from build123d import *

# Parameters (mm, degrees)
F0_W      = 5
F0_H      = 20
F1_DEPTH  = 35
F2_W      = 90
F2_H      = 25
F3_DEPTH  = 79.8669262783
F4_W      = 20
F4_H      = 35.1404882967
F5_DEPTH  = 5
F6_W      = 60
F6_H      = 25
F7_DEPTH  = 8.9178062806
F8_W      = 8.9168062806
F8_H      = 25
F9_DEPTH  = 12.5
F10_W     = 0.6563552694
F10_H     = 25
F11_DEPTH = 5
F12_W     = 7.5
F12_H     = 10
F13_DEPTH = 10


with BuildPart() as f1:
    # F0 (on Top) → F1 (new body)
    with BuildSketch(Plane.XY):
        Polygon((1.4652782414, 46.6247905791), (-88.5347217586, 60), (-88.5347217586, 40), (-88.5347217586, 0), (-88.5347217586, -20), (1.4652782414, -13.3752094209), align=None)
        with Locations((-91.0347217586, 50)):
            Rectangle(F0_W, F0_H)
        with Locations((-91.0347217586, -10)):
            Rectangle(F0_W, F0_H)
    extrude(amount=F1_DEPTH)

    # F2 (on face) → F3 (cut, through all)
    with BuildSketch(Plane(origin=(6.8110049505, 45.8303437542, 0), x_dir=(-0.9891366412, 0.1469989969, 0), z_dir=(0.1469989969, 0.9891366412, 0))):
        with Locations((50.404437048, 17.5)):
            Rectangle(F2_W, F2_H)
    extrude(amount=-F3_DEPTH, mode=Mode.SUBTRACT)

    # F4 (on face) → F5 (join)
    with BuildSketch(Plane(origin=(-93.5347217586, 0, 0), x_dir=(0, -1, 0), z_dir=(-1, 0, 0))):
        with Locations((10, 17.5702441484)):
            Rectangle(F4_W, F4_H)
    extrude(amount=-F5_DEPTH)

    # F6 (on face) → F7 (cut, through all)
    with BuildSketch(Plane.YZ.offset(1.4652782414)):
        with Locations((16.6247905791, 17.5)):
            Rectangle(F6_W, F6_H)
    extrude(amount=-F7_DEPTH, mode=Mode.SUBTRACT)

    # F8 (on face) → F9 (cut, symmetric)
    with BuildSketch(Plane(origin=(0, -13.3752094209, 0), x_dir=(-1, 0, 0), z_dir=(0, 1, 0))):
        with Locations((2.9931248989, 17.5)):
            Rectangle(F8_W, F8_H)
    extrude(amount=F9_DEPTH, both=True, mode=Mode.SUBTRACT)

    # F10 (on face) → F11 (cut, symmetric)
    with BuildSketch(Plane.YZ.offset(-7.4515280392)):
        with Locations((-13.7033870556, 17.5)):
            Rectangle(F10_W, F10_H)
    extrude(amount=F11_DEPTH, both=True, mode=Mode.SUBTRACT)

    # F12 (on face) → F13 (join)
    with BuildSketch(Plane.XY.offset(35)):
        with Locations((-64.7847217586, 25)):
            Rectangle(F12_W, F12_H)
    extrude(amount=F13_DEPTH)


solid = f1.part
The model under review builds one solid part; all positions refer to its coordinate system, in mm. A direction names the side the tool comes from. Round coordinates to 2 decimals unless told otherwise and drop trailing zeros. Write each loop counter-clockwise with the first axis right and the second up, starting at its lowest first coordinate (ties: lowest second). Pieces come first, ordered by that corner, then holes. Notation, with made-up numbers: M 9.25,80.5 L 45.25,80.5 A24 ccw 45.25,114.5 Z; hole C 68.25,55 d10. An arc over 180 degrees is marked long. Use a Markdown table: item, result. Add a question column.
Q1. Machinability: for faces 5 (the face through (-93.535, -10, 17)), 6 (the face through (-88.535, 20, 32)), 7 (the face through (-61.035, 25, 40)), which of the approach directions +Z, -Z, +X, -X, +Y, -Y give a long, thin tool a straight path to every point of the face, cutting with its end or side? Answer none if there is none.
Q2. We need section D-D, the plane y = -10. State the section outline as (x, z) points.
Q3. To check wall thickness, follow line 1 (Z direction, x = -15.5, y = -0.5); line 2 (X direction, y = 26.5, z = 42.5); line 3 (X direction, y = -6, z = 19). State the ranges of each line that lie inside material, in increasing order.
Q4. The part is to be moulded in two halves that separate along Z. For faces 1 (the face through (-88.535, -10, 18)), 2 (the face through (-89.01, 50.07, 17.33)), 3 (the face through (-91, -10, 35.14)), 4 (the face through (-68.535, 25, 40)), say which applies: pulls with the +Z half, pulls with the -Z half, needs draft (parallel to the pull), parting line crosses it, or undercut.
Q5. We need section C-C, the plane x = -5. State the section outline as (y, z) points.
Q6. We need section A-A, the plane y = 2. State the section outline as (x, z) points, plus the area to 3 significant figures.
Q7. Insertion check: pin 1 (2 mm diameter, centred on x = -64.5, z = 39.5, fed in from +Y); pin 2 (5 mm diameter, centred on y = 25.5, z = 42, fed in from +X); pin 3 (1 mm diameter, centred on x = -15.5, y = 46.5, fed in from +Z); pin 4 (1.5 mm diameter, centred on x = -15, z = 6, fed in from -Y). Each pin has a flat end and moves straight along its axis. Give the tip position at first contact, or say it passes through.
Findings below:
| question | item | result |
|---|---|---|
| 1 | face 5 | +Z, -Z, -X, +Y, -Y |
| 1 | face 6 | +Z, -Z, -X |
| 1 | face 7 | +Z, +X, +Y, -Y |
| 2 | outline | M -93.53,0 L 1.47,0 L 1.47,5 L -88.53,5 L -88.53,30 L 1.47,30 L 1.47,35 L -88.53,35 L -88.53,35.14 L -93.53,35.14 Z |
| 3 | line 1 | z = 0 to 5, 30 to 35 |
| 3 | line 2 | x = -68.53 to -61.03 |
| 3 | line 3 | x = -93.53 to -88.53 |
| 4 | face 1 | undercut |
| 4 | face 2 | undercut |
| 4 | face 3 | pulls with the +Z half |
| 4 | face 4 | needs draft |
| 5 | outline | M -13.85,0 L 47.59,0 L 47.59,5 L -13.85,5 Z; M -13.85,30 L 47.59,30 L 47.59,35 L -13.85,35 Z |
| 6 | outline | M -88.53,0 L 1.47,0 L 1.47,5 L -88.53,5 Z; M -88.53,30 L 1.47,30 L 1.47,35 L -88.53,35 Z |
| 6 | area | 900 mm² |
| 7 | pin 1 | stops at y = 30 |
| 7 | pin 2 | stops at x = -61.03 |
| 7 | pin 3 | stops at z = 35 |
| 7 | pin 4 | passes through |
